Geometry: final body of the model. Coordinates: model frame, mm. A direction names the side the tool comes from. Coordinates: 2 decimals unless noted, no trailing zeros. Write each loop counter-clockwise with the first axis right and the second up, starting at its lowest first coordinate (ties: lowest second). Pieces come first, ordered by that corner, then holes. Notation, with made-up numbers: (39, -19) -> (78, -19) arc R12 ccw to (78, -6) -> close; hole circle Ø7 at (-4, 68.5). An arc over 180 degrees is marked (long way). One line per item, written item: value.
Autodesk Inventor part; units mm, degrees
ref_plane "YZ Plane" through (0, 0, 0) normal (1, 0, 0) x (0, 1, 0)
ref_plane "XZ Plane" through (0, 0, 0) normal (0, 1, 0) x (-1, 0, 0)
ref_plane "XY Plane" through (0, 0, 0) normal (0, 0, 1) x (1, 0, 0)
sketch "Эскиз1" plane through (0, 0, 0) normal (0, 1, 0) x (-1, 0, 0)
  line L0 (0, 0) -> (40, 0)
  line L1 (40, 0) -> (40, 60)
  line L2 (40, 60) -> (0, 60)
  line L3 (0, 60) -> (0, 0)
  dimension "d0" = 60
  dimension "d1" = 40
extrude "Выдавливание1" add sketch "Эскиз1" along normal blind 190
sketch "Эскиз2" plane through (0, 190, 0) normal (0, 1, 0) x (1, 0, 0)
  line L0 (-35, -5) -> (-5, -5)
  line L1 (-5, -5) -> (-5, -55)
  line L2 (-5, -55) -> (-35, -55)
  line L3 (-35, -55) -> (-35, -5)
  line L4 (-40, 0) -> (-40, -60)
  line L5 (0, -60) -> (0, 0)
  line L6 (0, 0) -> (-40, 0)
  line L7 (-40, -60) -> (0, -60)
  dimension "d4" = 5
  dimension "d5" = 5
  dimension "d6" = 5
  dimension "d7" = 5
extrude "Выдавливание2" cut sketch "Эскиз2" against normal through all contours L0 L1 L2 L3
sketch "Эскиз3" plane through (-40, 0, 60) normal (0, 0, 1) x (1, 0, 0)
  point P0 (40, 0)
sketch "Эскиз5" plane through (0, 190, 0) normal (0, 1, 0) x (1, 0, 0)
  line L0 (-5, -5) -> (-5, -55)
  line L1 (-5, -55) -> (-35, -55)
  line L2 (-35, -55) -> (-35, -5)
  line L3 (-35, -5) -> (-5, -5)
  line L4 (-40, 0) -> (-40, -60)
  line L5 (-40, -60) -> (0, -60)
  line L6 (0, -60) -> (0, 0)
  line L7 (0, 0) -> (-40, 0)
extrude "Выдавливание4" cut sketch "Эскиз5" against normal blind 45
equation "\"d5\" = d4"
equation "\"d6\" = d4"
equation "\"d7\" = d4"
properties part number "БРУС"
(1) Reachability of faces 1 (the flat face through (-20, 74, 5)), 2 (the flat face through (0, 71, 30)) from +Z, -Z, +X, -X, +Y, -Y: full face, straight path, thin tool, end or side. Return the list, or none.
Responses:
face 1: +Y, -Y
face 2: +Z, -Z, +X, +Y, -Y
(2) Line query: line 1 (Z direction, x = -21.5, y = 129); line 2 (X direction, y = 124, z = 26). Output: solid intervals per line, ascending. Write a range as [from, to].
Responses:
line 1: z = [0, 5], [55, 60]
line 2: x = [-40, -35], [-5, 0]
(3) Section A-A (z = 12). Return the cut outline in (x, y), then the cut area to 3 significant figures.
Responses:
outline: (-40, 0) -> (-35, 0) -> (-35, 145) -> (-40, 145) -> close; (-5, 0) -> (0, 0) -> (0, 145) -> (-5, 145) -> close
area: 1,450 mm2
(4) Section C-C (x = -15). Return the cut outline in (y, z).
Responses:
outline: (0, 0) -> (145, 0) -> (145, 5) -> (0, 5) -> close; (0, 55) -> (145, 55) -> (145, 60) -> (0, 60) -> close
(5) Section B-B (y = 9.5). Return the cut outline in (x, z).
Responses:
outline: (-40, 0) -> (0, 0) -> (0, 60) -> (-40, 60) -> close; hole (-35, 5) -> (-5, 5) -> (-5, 55) -> (-35, 55) -> close
(6) Pull-direction query (X, two-part tool) for faces 3 (the flat face through (-40, 71, 30)), 4 (the flat face through (-20, 74, 55)), 5 (the flat face through (-2, 0, 30)); classes: released by +X, released by -X, zero draft, split by the parting line, or undercut.
Responses:
face 3: released by -X
face 4: undercut
face 5: zero draft
